Can you work these out from the model? Positions are in its coordinate system, mm. Face numbers are marked on the shaded views. A direction names the side the tool comes from. Round coordinates to 2 decimals unless told otherwise and drop trailing zeros. Loops run counter-clockwise (first coordinate to the right, second up) from the corner with the lowest first, then second, coordinate; pieces in that order, holes last. Notation, with made-up numbers: M 53,41.5 L 102,41.5 A14 ccw 102,45.5 Z; hole C -38.75,58 d6. An arc over 180 degrees is marked long. Use a Markdown table: item, result. Add a question column.
```python
from build123d import *

# Parameters (mm, degrees)
STRAP_DEPTH        = 4
EAR_HOLES_M4_START = -0.5
SKETCH2_R          = 2.25
EAR_HOLES_M4_DEPTH = 5


with BuildPart() as part:
    # Sketch1 → Strap (new, symmetric)
    with BuildSketch(Plane(origin=(0, 0, 0), x_dir=(0, 0, -1), z_dir=(1, 0, 0))):
        Polygon((-36.15, 0), (-18.15, 0), (-18.15, 28.3), (18.15, 28.3), (18.15, 0), (36.15, 0), (36.15, 4), (22.15, 4), (22.15, 32.3), (-22.15, 32.3), (-22.15, 4), (-36.15, 4), align=None)
    extrude(amount=STRAP_DEPTH, both=True)

    # Sketch2 → Ear_Holes_M4 (cut)
    with BuildSketch(Plane(origin=(0, 0, 0), x_dir=(1, 0, 0), z_dir=(0, 1, 0)).offset(EAR_HOLES_M4_START)):
        with Locations(Location((0, 29.15, 0), (0, 0, 90))):
            Circle(SKETCH2_R)
        with Locations(Location((0, -29.15, 0), (0, 0, 90))):
            Circle(SKETCH2_R)
    extrude(amount=EAR_HOLES_M4_DEPTH, mode=Mode.SUBTRACT)


solid = part.part
```
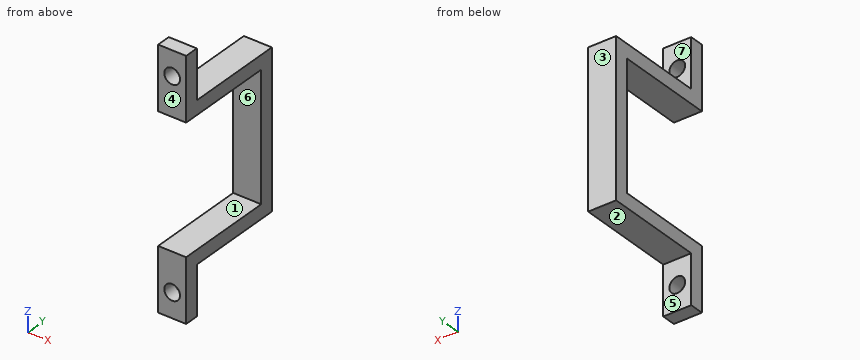
(1) If I drill on probe 1 along Z at (x, y) = (2.25, 24.5); probe 2 along X at (y, z) = (1, 29) (3 decimals); probe 3 along Y at (x, z) = (3.25, -6.5), over which ranges is the centre line in solid material (lowest first)? Write a range as [from, to].
(2) On a 3-axis mill with a long thin cutter (end or side, diameter ignored), from which of +Z, -Z, +X, -X, +Y, -Y can I reach the whole of each face in a straight line? I mean the marked faces 4, 5, 6 and 7. Say none if no direction works.
(3) I'm going to push flat-ended pins straight in: pin 1 (2 mm diameter, centred on x = 0.5, y = 11.5, fed in from +Z); pin 2 (1.5 mm diameter, centred on x = -0.5, z = 3.5, fed in from -Y); pin 3 (1.5 mm diameter, centred on x = 1.5, y = 24, fed in from -Z); pin 4 (12 mm diameter, centred on y = 16.5, z = 25, fed in from +X). Where does each tip first touch, or does it pass through?
(4) Suppose I cut it at D-D on z = -9. List the corners of the cut face in (x, y) for me.
(5) Suppose I cut it at A-A on y = 7. List the corners of the cut face in (x, z) for me.
(6) Suppose I cut it at C-C on z = 29.15. List the corners of the cut face in (x, y) for me, and give its area (3 significant figures).
(7) Thinking about a two-plate mould opening in Z: for the marked faces 1, 2 and 3, which applies, released by +Z, released by -Z, zero draft, split by the parting line, or undercut?
(8) Suppose I cut it at B-B on x = 0. List the corners of the cut face in (y, z) for me, and give its area (3 significant figures).
Results below:
| question | item | result |
|---|---|---|
| 1 | probe 1 | z = [-22.15, -18.15], [18.15, 22.15] |
| 1 | probe 2 | x = [-4, -2.245], [2.245, 4] |
| 1 | probe 3 | y = [28.3, 32.3] |
| 2 | face 4 | +Z, -Z, +X, -X, -Y |
| 2 | face 5 | -Z, +X, -X, +Y |
| 2 | face 6 | +X, -X, -Y |
| 2 | face 7 | +Z, +X, -X, +Y |
| 3 | pin 1 | stops at z = 22.15 |
| 3 | pin 2 | stops at y = 28.3 |
| 3 | pin 3 | stops at z = -22.15 |
| 3 | pin 4 | stops at x = 4 |
| 4 | outline | M -4,28.3 L 4,28.3 L 4,32.3 L -4,32.3 Z |
| 5 | outline | M -4,-22.15 L 4,-22.15 L 4,-18.15 L -4,-18.15 Z; M -4,18.15 L 4,18.15 L 4,22.15 L -4,22.15 Z |
| 6 | outline | M -4,0 L -2.25,0 L -2.25,4 L -4,4 Z; M 2.25,0 L 4,0 L 4,4 L 2.25,4 Z |
| 6 | area | 14.0 mm² |
| 7 | face 1 | undercut |
| 7 | face 2 | released by -Z |
| 7 | face 3 | zero draft |
| 8 | outline | M 0,-36.15 L 4,-36.15 L 4,-31.4 L 0,-31.4 Z; M 0,-26.9 L 4,-26.9 L 4,-22.15 L 32.3,-22.15 L 32.3,22.15 L 4,22.15 L 4,26.9 L 0,26.9 L 0,18.15 L 28.3,18.15 L 28.3,-18.15 L 0,-18.15 Z; M 0,31.4 L 4,31.4 L 4,36.15 L 0,36.15 Z |
| 8 | area | 480 mm² |
